from build123d import *

# Parameters (mm, degrees)
SKETCH_1_R          = 100
EXTRUDE_1_DEPTH     = 3
SKETCH_2_R          = 2
CUT_EXTRUDE_1_DEPTH = 10
SKETCH_4_W          = 70
SKETCH_4_H          = 35
CUT_EXTRUDE_2_DEPTH = 10
SKETCH_5_R          = 2
CUT_EXTRUDE_3_DEPTH = 10
SKETCH_6_W          = 3
SKETCH_6_H          = 25
EXTRUDE_2_DEPTH     = 25
SKETCH_7_R          = 1
CUT_EXTRUDE_4_DEPTH = 30
CHAMFER_1_SIZE      = 10
CHAMFER_2_SIZE      = 10
CHAMFER_3_SIZE      = 5
SKETCH_11_W         = 2
SKETCH_11_H         = 30
CUT_EXTRUDE_5_DEPTH = 30
SKETCH_12_R         = 1.5
SKETCH_12_R_2       = 1.364499713
CUT_EXTRUDE_6_DEPTH = 10
SKETCH_13_W         = 2.5
SKETCH_13_H         = 30
CUT_EXTRUDE_7_DEPTH = 10
SKETCH_14_RX        = 17.045359967
SKETCH_14_RY        = 11.452351228
CUT_EXTRUDE_8_DEPTH = 10


with BuildPart() as part:
    # Эскиз1 → Бобышка-Вытянуть1 (new body)
    with BuildSketch(Plane(origin=(0, 0, 0), x_dir=(1, 0, 0), z_dir=(0, 1, 0))):
        with Locations(Location((0, 0, 0), (0, 0, 270))):
            Circle(SKETCH_1_R)
    extrude(amount=EXTRUDE_1_DEPTH)

    # Эскиз2 → Вырез-Вытянуть1 (cut)
    with BuildSketch(Plane(origin=(0, 3, 0), x_dir=(1, 0, 0), z_dir=(0, 1, 0))):
        with Locations(Location((85, 0, 0), (0, 0, 270))):
            Circle(SKETCH_2_R)
        with Locations(Location((65.113777665, -54.636946823, 0), (0, 0, 270))):
            Circle(SKETCH_2_R)
        with Locations(Location((14.760095102, -83.708659006, 0), (0, 0, 270))):
            Circle(SKETCH_2_R)
        with Locations(Location((-42.5, -73.612159322, 0), (0, 0, 270))):
            Circle(SKETCH_2_R)
        with Locations(Location((-79.873872767, -29.071712183, 0), (0, 0, 270))):
            Circle(SKETCH_2_R)
        with Locations(Location((-79.873872767, 29.071712183, 0), (0, 0, 270))):
            Circle(SKETCH_2_R)
        with Locations(Location((-42.5, 73.612159322, 0), (0, 0, 270))):
            Circle(SKETCH_2_R)
        with Locations(Location((14.760095102, 83.708659006, 0), (0, 0, 270))):
            Circle(SKETCH_2_R)
        with Locations(Location((65.113777665, 54.636946823, 0), (0, 0, 270))):
            Circle(SKETCH_2_R)
    extrude(amount=-CUT_EXTRUDE_1_DEPTH, mode=Mode.SUBTRACT)

    # Эскиз4 → Вырез-Вытянуть2 (cut)
    with BuildSketch(Plane(origin=(0, 3, 0), x_dir=(1, 0, 0), z_dir=(0, 1, 0))):
        with Locations((-52, -87.543045262)):
            Rectangle(SKETCH_4_W, SKETCH_4_H)
        with Locations((-52, 87.543045262)):
            Rectangle(SKETCH_4_W, SKETCH_4_H)
    extrude(amount=-CUT_EXTRUDE_2_DEPTH, mode=Mode.SUBTRACT)

    # Эскиз5 → Вырез-Вытянуть3 (cut)
    with BuildSketch(Plane(origin=(0, 3, 0), x_dir=(1, 0, 0), z_dir=(0, 1, 0))):
        with Locations(Location((39.936936383, -75.033599889, 0), (0, 0, 270))):
            Circle(SKETCH_5_R)
        with Locations(Location((39.936936383, 75.033599889, 0), (0, 0, 270))):
            Circle(SKETCH_5_R)
        with Locations(Location((-65, 54.772255751, 0), (0, 0, 270))):
            Circle(SKETCH_5_R)
        with Locations(Location((-65, -54.772255751, 0), (0, 0, 270))):
            Circle(SKETCH_5_R)
    extrude(amount=-CUT_EXTRUDE_3_DEPTH, mode=Mode.SUBTRACT)

    # Эскиз6 → Бобышка-Вытянуть2 (add)
    with BuildSketch(Plane.XZ):
        with Locations((-88.5, 0)):
            Rectangle(SKETCH_6_W, SKETCH_6_H)
    extrude(amount=EXTRUDE_2_DEPTH)

    # Эскиз7 → Вырез-Вытянуть4 (cut)
    with BuildSketch(Plane.ZY.offset(90)):
        with Locations((-10, -22.5)):
            Circle(SKETCH_7_R)
        with Locations((10, -22.5)):
            Circle(SKETCH_7_R)
        with Locations((-10, -8.5)):
            Circle(SKETCH_7_R)
        with Locations((10, -8.5)):
            Circle(SKETCH_7_R)
    extrude(amount=-CUT_EXTRUDE_4_DEPTH, mode=Mode.SUBTRACT)

    # Фаска1
    chamfer_1_edges = [part.edges().sort_by_distance(p)[0] for p in [
        (-88.5, 0, -12.5),
    ]]
    chamfer(chamfer_1_edges, length=CHAMFER_1_SIZE)

    # Фаска2
    chamfer_2_edges = [part.edges().sort_by_distance(p)[0] for p in [
        (-88.5, 0, 12.5),
    ]]
    chamfer(chamfer_2_edges, length=CHAMFER_2_SIZE)

    # Фаска3
    chamfer_3_edges = [part.edges().sort_by_distance(p)[0] for p in [
        (-87, 0, 0),
    ]]
    chamfer(chamfer_3_edges, length=CHAMFER_3_SIZE)

    # Эскиз11 → Вырез-Вытянуть5 (cut)
    with BuildSketch(Plane.XZ):
        with Locations((-91, 0.438486228)):
            Rectangle(SKETCH_11_W, SKETCH_11_H)
    extrude(amount=-CUT_EXTRUDE_5_DEPTH, mode=Mode.SUBTRACT)

    # Эскиз12 → Вырез-Вытянуть6 (cut)
    with BuildSketch(Plane.XZ):
        with Locations(Location((1.260095102, -29.5, 0), (0, 0, 270))):
            Circle(SKETCH_12_R)
        with Locations(Location((1.260095102, 29.5, 0), (0, 0, 270))):
            Circle(SKETCH_12_R)
        with Locations(Location((28.260095102, -29.5, 0), (0, 0, 270))):
            Circle(SKETCH_12_R)
        with Locations(Location((28.260095102, 29.5, 0), (0, 0, 270))):
            Circle(SKETCH_12_R)
        with Locations(Location((-70.688878581, 40, 0), (0, 0, 270))):
            Circle(SKETCH_12_R_2)
        with Locations(Location((-27.73782315, 40.032744033, 0), (0, 0, 270))):
            Circle(SKETCH_12_R)
        with Locations(Location((-21.688878581, 40, 0), (0, 0, 270))):
            Circle(SKETCH_12_R_2)
        with Locations(Location((-21.688878581, -18.085512482, 0), (0, 0, 270))):
            Circle(SKETCH_12_R_2)
        with Locations(Location((-64.489792506, -17.736958402, 0), (0, 0, 270))):
            Circle(SKETCH_12_R)
        with Locations(Location((-70.688878581, -18.085512482, 0), (0, 0, 270))):
            Circle(SKETCH_12_R_2)
    extrude(amount=-CUT_EXTRUDE_6_DEPTH, mode=Mode.SUBTRACT)

    # Эскиз13 → Вырез-Вытянуть7 (cut)
    with BuildSketch(Plane.XZ):
        with Locations((57.794423637, 0)):
            Rectangle(SKETCH_13_W, SKETCH_13_H)
        with Locations((71.075546462, 0)):
            Rectangle(SKETCH_13_W, SKETCH_13_H)
    extrude(amount=-CUT_EXTRUDE_7_DEPTH, mode=Mode.SUBTRACT)

    # Эскиз14 → Вырез-Вытянуть8 (cut)
    with BuildSketch(Plane.XZ):
        with Locations(Location((17.045359967, 53.266749896), (0, 0, 180))):
            Ellipse(SKETCH_14_RX, SKETCH_14_RY)
        with Locations(Location((17.045359967, -53.266749896), (0, 0, 180))):
            Ellipse(SKETCH_14_RX, SKETCH_14_RY)
    extrude(amount=-CUT_EXTRUDE_8_DEPTH, mode=Mode.SUBTRACT)


solid = part.part
Can you work these out from the model? Positions are in its coordinate system, mm. A direction names the side the tool comes from. Give positions to 0.01 mm unless a question says otherwise; leave off trailing zeros. Loops run counter-clockwise (first coordinate to the right, second up) from the corner with the lowest first, then second, coordinate; pieces in that order, holes last. Notation, with made-up numbers: (41, -2) - (93, -2) arc R20 ccw to (93, 24) - close; hole circle Ø10 at (30.5, 11.5). An arc over 180 degrees is marked (long way). One line per item, written item: value.
(1) If we section it at A-A, the plane y = -18.5: List the corners of the cut face in (x, z) for me, plus the area to 3 significant figures.
Verdict:
outline: (-90, -12.5) - (-87, -12.5) - (-87, 12.5) - (-90, 12.5) - close
area: 75.0 mm^2
(2) I'm going to push flat-ended pins straight in: pin 1 (4 mm diameter, centred on x = -27.74, z = 40.03, fed in from +Y); pin 2 (6.5 mm diameter, centred on x = 39.94, z = 75.03, fed in from -Y); pin 3 (2.5 mm diameter, centred on x = -45, y = 1, fed in from +Z); pin 4 (3 mm diameter, centred on y = -22.5, z = 10, fed in from +X). Where does each tip first touch, or does it pass through?
Verdict:
pin 1: y = 3
pin 2: y = 0
pin 3: z = 70.04
pin 4: x = -87
(3) If we section it at B-B, the plane x = -3.5: List the corners of the cut face in (y, z) for me.
Verdict:
outline: (0, -99.94) - (3, -99.94) - (3, 99.94) - (0, 99.94) - close
(4) On a 3-axis mill with a long thin cutter (end or side, diameter ignored), from which of +Z, -Z, +X, -X, +Y, -Y can I reach the whole of each face in a straight line? I mean faces 1 (the face through (-87, -15, 0)), 2 (the face through (-87.8, -4, 18.5)). Say none if no direction works.
Verdict:
face 1: +Z, -Z, +X, -Y
face 2: +Z, +X, -X, -Y
(5) I need wall thicknesses on line 1 along Y through (x, z) = (-89.15, -10); line 2 along X through (y, z) = (0.85, 40); line 3 along X through (y, z) = (2.05, -29.5). Which ranges of each line are inside material? Lowest first, please.
Verdict:
line 1: -25 to -23.5, -21.5 to -9.5, -7.5 to 3
line 2: -91.65 to -72.05, -69.32 to -29.24, -26.24 to -23.05, -20.32 to 91.65
line 3: -95.55 to -81.83, -77.92 to -0.24, 2.76 to 26.76, 29.76 to 95.55
